Check sheet for the modelled part. Datum: model origin and axes. Units: mm. A direction names the side the tool comes from. Round coordinates to 2 decimals unless told otherwise and drop trailing zeros. Loops run counter-clockwise (first coordinate to the right, second up) from the corner with the lowest first, then second, coordinate; pieces in that order, holes last. Notation, with made-up numbers: (78.5, 70.25) - (136.5, 70.25) arc R19 ccw to (136.5, 78.25) - close; hole circle Ø10 at (-25, -7). An arc over 180 degrees is marked (long way). Return JSON: item names as keys, results as strings.
Autodesk Inventor part; units mm, degrees
ref_plane "YZ Plane" through (0, 0, 0) normal (1, 0, 0) x (0, 1, 0)
ref_plane "XZ Plane" through (0, 0, 0) normal (0, 1, 0) x (-1, 0, 0)
ref_plane "XY Plane" through (0, 0, 0) normal (0, 0, 1) x (1, 0, 0)
sketch "Sketch1" plane through (0, 0, 0) normal (0, 0, 1) x (1, 0, 0)
  line L0 (100, 0) -> (700, 0)
  line L1 (800, -100) -> (800, -700)
  line L2 (700, -800) -> (100, -800)
  line L3 (0, -700) -> (0, -100)
  arc A0 (2, 0) -> (0, -2) centre (2, -2) ccw
  arc A1 (800, -100) -> (700, 0) centre (700, -100) ccw
  arc A2 (100, 0) -> (0, -100) centre (100, -100) ccw
  arc A3 (0, -700) -> (100, -800) centre (100, -700) ccw
  arc A4 (700, -800) -> (800, -700) centre (700, -700) ccw
  point P0 (0, 0)
  point P1 (800, -800)
  point P2 (0, -800)
  dimension "d0" = 800
  dimension "d1" = 800
  dimension "d2" = 2
  dimension "d3" = 100
extrude "Extrusion1" add sketch "Sketch1" along normal blind 800
sketch "Sketch2" plane through (0, -700, 0) normal (-1, 0, 0) x (0, 0, 1)
  line L0 (250, 450) -> (550, 450)
  line L1 (550, 450) -> (550, 300)
  line L2 (550, 300) -> (250, 300)
  line L3 (250, 300) -> (250, 450)
  line L4 (0, 700) -> (800, 700)
  line L5 (0, -100) -> (800, -100)
  line L6 (800, 600) -> (800, 0)
  line L7 (0, 600) -> (0, 0)
  dimension "d6" = 300
  dimension "d7" = 150
  dimension "d8" = 250
  dimension "d9" = 400
  dimension "d10" = 250
  dimension "d11" = 250
extrude "Extrusion2" cut sketch "Sketch2" against normal blind 200
fillet "Fillet1" radius 100 16 edges at (29.2893, -770.7107, 0) (400, -800, 0) (770.7107, -770.7107, 0) (800, -400, 0) (770.7107, -29.2893, 0) (400, 0, 0) (29.2893, -29.2893, 0) (0, -400, 0) (29.2893, -770.7107, 800) (400, -800, 800) (770.7107, -770.7107, 800) (800, -400, 800) (770.7107, -29.2893, 800) (400, 0, 800) (29.2893, -29.2893, 800) (0, -400, 800)
sketch "Sketch3" plane through (100, -800, 700) normal (0, -1, 0) x (1, 0, 0)
  circle A0 centre (300, -298.1465) radius 275
  line L0 (-100, -600) -> (-100, 0)
  line L1 (700, -600) -> (700, 0)
  point P0 (-100, -700)
  dimension "d15" = 550
  dimension "d16" = 400
  dimension "d17" = 400
extrude "Extrusion3" cut sketch "Sketch3" against normal blind 700
sketch "Sketch4" plane through (0, -700, 700) normal (-1, 0, 0) x (0, 0, 1)
  line L0 (-560.17, 235.0251) -> (-460.17, 235.0251)
  line L1 (-460.17, 235.0251) -> (-460.17, 205.0251)
  line L2 (-460.17, 205.0251) -> (-560.17, 205.0251)
  line L3 (-560.17, 205.0251) -> (-560.17, 235.0251)
  point P0 (-700, 700)
  dimension "d20" = 100
  dimension "d21" = 30
extrude "Extrusion4" cut sketch "Sketch4" against normal blind 200
sketch "Sketch5" plane through (800, -700, 700) normal (1, 0, 0) x (0, 0, -1)
  line L0 (129.5986, 209.4371) -> (429.5986, 209.4371) construction
  line L1 (129.5986, 159.4371) -> (429.5986, 159.4371)
  line L2 (429.5986, 259.4371) -> (129.5986, 259.4371)
  arc A0 (129.5986, 259.4371) -> (129.5986, 159.4371) centre (129.5986, 209.4371) ccw
  arc A1 (429.5986, 159.4371) -> (429.5986, 259.4371) centre (429.5986, 209.4371) ccw
  point P0 (700, 700)
  point P1 (279.5986, 209.4371)
  dimension "d24" = 300
  dimension "d25" = 100
extrude "Extrusion5" cut sketch "Sketch5" against normal blind 200
properties part number "Head_prototype2"
Q1. Sectioned sample at C-C (x = 400). Enter the section's corners in (y, z).
Answer key:
{"outline": "(-800, 100) arc R100 ccw to (-700, 0) - (-100, 0) arc R100 ccw to (0, 100) - (0, 700) arc R100 ccw to (-100, 800) - (-700, 800) arc R100 ccw to (-800, 700) - (-800, 676.85) - (-100, 676.85) - (-100, 126.85) - (-800, 126.85) - close"}
Q2. Sectioned sample at D-D (y = -572). Enter the section's corners in (x, z), plus the area to 3 significant figures.
Answer key:
{"outline": "(0, 100) arc R100 ccw to (100, 0) - (700, 0) arc R100 ccw to (800, 100) - (800, 700) arc R100 ccw to (700, 800) - (100, 800) arc R100 ccw to (0, 700) - close; hole circle Ø550 at (400, 401.85)", "area": "394,000 mm²"}
Q3. Sectioned sample at B-B (y = -267.5). Enter the section's corners in (x, z), plus the area to 3 significant figures.
Answer key:
{"outline": "(0, 100) arc R100 ccw to (100, 0) - (700, 0) arc R100 ccw to (800, 100) - (800, 700) arc R100 ccw to (700, 800) - (100, 800) arc R100 ccw to (0, 700) - (0, 550) - (168.32, 550) arc R275 cw (long way) to (170.73, 250) - (0, 250) - close", "area": "352,000 mm²"}
Q4. Scan lines: probe 1 along Z at (x, y) = (392, -533.5); probe 2 along Z at (x, y) = (400, -370.5); probe 3 along X at (y, z) = (-661, 397.5). Record each from-to range of solid material in increasing order. Write a range as [from, to].
Answer key:
{"probe 1": "z = [0, 126.97], [676.74, 800]", "probe 2": "z = [0, 126.85], [676.85, 800]", "probe 3": "x = [0, 125.03], [674.97, 800]"}
Q5. Draft check along Y on faces 4 (the face through (200, -480, 176)), 5 (the face through (30.071, -771.484, 395.8)), 6 (the face through (800, -396, 396)). Enter one of: released by +Y, released by -Y, zero draft, split by the parting line, or undercut.
Answer key:
{"face 4": "undercut", "face 5": "released by -Y", "face 6": "zero draft"}
Q6. Sectioned sample at A-A (z = 361). Enter the section's corners in (x, y).
Answer key:
{"outline": "(0, -700) arc R100 ccw to (100, -800) - (128.05, -800) - (128.05, -400) - (0, -400) - close; (0, -250) - (128.05, -250) - (128.05, -100) - (671.95, -100) - (671.95, -440.56) - (800, -440.56) - (800, -100) arc R100 ccw to (700, 0) - (100, 0) arc R100 ccw to (0, -100) - close; (671.95, -800) - (700, -800) arc R100 ccw to (800, -700) - (800, -540.56) - (671.95, -540.56) - close"}
Q7. Depth check by flat-ended pin: P1, Ø9, axis at y = -473, z = 191, coming from the -X side; P2, Ø10, axis at x = 381, z = 381.5, coming from the -Y side; P3, Ø24, axis at x = 98.5, y = -485, coming from the +Z side; P4, Ø4, axis at x = 709, y = -606.5, coming from the +Z side. Enter the tip coordinate at first touch or a pass-through.
Answer key:
{"P1": "stops at x = 200", "P2": "stops at y = -100", "P3": "stops at z = 800", "P4": "stops at z = 799.75"}
Q8. Tool access check on faces 1 (the face through (83, -324, 550)), 2 (the face through (88, -480, 239.83)), 3 (the face through (600, -490, 602)). Record the directions out of +Z, -Z, +X, -X, +Y, -Y that give a thin tool (end or side, any length) a straight path to the whole face; none if there is none.
Answer key:
{"face 1": "-X", "face 2": "+X, -X", "face 3": "+X"}
